from build123d import *

# Parameters (mm, degrees)
CROQUIS1_R              = 100
SALIENTE_EXTRUIR1_DEPTH = 3
CROQUIS3_R              = 110
CORTAR_EXTRUIR1_DEPTH   = 3
REDONDEO1_R             = 10
CORTAR_EXTRUIR2_DEPTH   = 142.453172607
CROQUIS5_R              = 1.5
CORTAR_EXTRUIR3_DEPTH   = 10
CROQUIS6_R              = 2
CORTAR_EXTRUIR4_DEPTH   = 142.453172607


with BuildPart() as part:
    # Croquis1 → Saliente-Extruir1 (new body)
    with BuildSketch(Plane.XY):
        Circle(CROQUIS1_R)
    extrude(amount=SALIENTE_EXTRUIR1_DEPTH)

    # Croquis3 → Cortar-Extruir1 (cut)
    with BuildSketch(Plane.XY.offset(3)):
        with Locations((190, 0)):
            Circle(CROQUIS3_R)
    extrude(amount=-CORTAR_EXTRUIR1_DEPTH, mode=Mode.SUBTRACT)

    # Redondeo1
    redondeo1_edges = [part.edges().sort_by_distance(p)[0] for p in [
        (89.473684211, -44.659375654, 1.5),
        (89.473684211, 44.659375654, 1.5),
    ]]
    fillet(redondeo1_edges, radius=REDONDEO1_R)

    # Croquis4 → Cortar-Extruir2 (cut, through all)
    with BuildSketch(Plane.XY.offset(3)):
        Polygon((-83.792153571, -57.629202667), (-57.629202667, -83.792153571), (-42.072853481, -68.235804385), (-45.290189335, -65.01846853), (-8.520636713, -28.248915908), (-28.248915908, -8.520636713), (-65.01846853, -45.290189335), (-68.235804385, -42.072853481), align=None)
        Polygon((-8.520636713, 31.077343033), (-28.248915908, 11.349063838), (-65.01846853, 48.11861646), (-68.235804385, 44.901280605), (-83.792153571, 60.457629791), (-57.629202667, 86.620580695), (-42.072853481, 71.064231509), (-45.290189335, 67.846895655), align=None)
        Polygon((31.077343033, 11.349063838), (11.349063838, 31.077343033), (48.11861646, 67.846895655), (44.901280605, 71.064231509), (60.457629791, 86.620580695), (86.620580695, 60.457629791), (71.064231509, 44.901280605), (67.846895655, 48.11861646), align=None)
        Polygon((11.349063838, -28.248915908), (31.077343033, -8.520636713), (67.846895655, -45.290189335), (71.064231509, -42.072853481), (86.620580695, -57.629202667), (60.457629791, -83.792153571), (44.901280605, -68.235804385), (48.11861646, -65.01846853), align=None)
    extrude(amount=-CORTAR_EXTRUIR2_DEPTH, mode=Mode.SUBTRACT)

    # Croquis5 → Cortar-Extruir3 (cut)
    with BuildSketch(Plane.XY.offset(3)):
        with Locations((-64.311361749, -40.340441867)):
            Circle(CROQUIS5_R)
        with Locations((-48.401459172, -24.43053929)):
            Circle(CROQUIS5_R)
        with Locations((-24.43053929, -48.401459172)):
            Circle(CROQUIS5_R)
        with Locations((-40.340441867, -64.311361749)):
            Circle(CROQUIS5_R)
        with Locations((-24.43053929, 51.229886297)):
            Circle(CROQUIS5_R)
        with Locations((-40.340441867, 67.139788874)):
            Circle(CROQUIS5_R)
        with Locations((-48.401459172, 27.258966415)):
            Circle(CROQUIS5_R)
        with Locations((-64.311361749, 43.168868991)):
            Circle(CROQUIS5_R)
        with Locations((51.229886297, 27.258966415)):
            Circle(CROQUIS5_R)
        with Locations((67.139788874, 43.168868991)):
            Circle(CROQUIS5_R)
        with Locations((27.258966415, 51.229886297)):
            Circle(CROQUIS5_R)
        with Locations((43.168868991, 67.139788874)):
            Circle(CROQUIS5_R)
        with Locations((27.258966415, -48.401459172)):
            Circle(CROQUIS5_R)
        with Locations((43.168868991, -64.311361749)):
            Circle(CROQUIS5_R)
        with Locations((51.229886297, -24.43053929)):
            Circle(CROQUIS5_R)
        with Locations((67.139788874, -40.340441867)):
            Circle(CROQUIS5_R)
    extrude(amount=-CORTAR_EXTRUIR3_DEPTH, mode=Mode.SUBTRACT)

    # Croquis6 → Cortar-Extruir4 (cut, through all)
    with BuildSketch(Plane(origin=(0, 0, 0), x_dir=(-1, 0, 0), z_dir=(0, 0, -1))):
        with Locations((-36.071652756, 84.633538668)):
            Circle(CROQUIS6_R)
        with Locations((34.338438835, 85.35145938)):
            Circle(CROQUIS6_R)
        with Locations((84.633538668, 36.071652756)):
            Circle(CROQUIS6_R)
        with Locations((85.35145938, -34.338438835)):
            Circle(CROQUIS6_R)
        with Locations((36.071652756, -84.633538668)):
            Circle(CROQUIS6_R)
        with Locations((-34.338438835, -85.35145938)):
            Circle(CROQUIS6_R)
    extrude(amount=-CORTAR_EXTRUIR4_DEPTH, mode=Mode.SUBTRACT)


solid = part.part
The listing builds one solid part. Answer for the finished solid, in the listing's coordinates (mm). A direction names the side the tool comes from. Coordinates: 2 decimals unless noted, no trailing zeros. Loops run counter-clockwise (first coordinate to the right, second up) from the corner with the lowest first, then second, coordinate; pieces in that order, holes last. Notation, with made-up numbers: (40, -9) -> (89, -9) arc R11 ccw to (89, 0) -> close; hole circle Ø9 at (-30, 73). An arc over 180 degrees is marked (long way). Write item = value, one per line. Start each with the question number.
1) A tool of negligible diameter and unlimited length cuts with its end or side. For faces 4 (the face through (-46.38, -26.65, 1.52)), 5 (the face through (-75.303, -49.14, 1.521)), 6 (the face through (-74.73, 51.396, 1.521)), from which of +Z, -Z, +X, -X, +Y, -Y can it reach the whole face along a straight path? Write none if from no direction.
2) Straight lines are drawn through the part: line 1 (X direction, y = 11.5, z = 2.05); line 2 (Y direction, x = 14, z = 1); line 3 (Y direction, x = 31.5, z = 2.7). For each, find the intervals that lie inside material, in ascending order. Write a range as from..to.
3) A cutting plane is placed at D-D (y = -1.5). Give the vertices of the cut face in (x, z).
4) A cutting plane is placed at A-A (x = 14). Give the vertices of the cut face in (y, z), then the cut area to 3 significant figures.
5) A cutting plane is placed at C-C (z = 2.3). Count the separate pieces of the cut face and the enclosed holes in it, then the cut area to 3 significant figures.
6) The mould has two halves that part along X. Classify faces 1 (the face through (84.96, 52.74, 1.48)), 2 (the face through (-99.983, 1.869, 1.479)), 3 (the face through (29.476, 49.205, 1.521)): released by +X, released by -X, zero draft, split by the parting line, or undercut.
7) A cutting plane is placed at B-B (y = -60). Give the vertices of the cut face in (x, z).
Responses:
q1.face_4 = +Z, -Z
q1.face_5 = +Z, -Z, -Y
q1.face_6 = +Z, -Z, +Y
q2.line_1 = -99.34..-28.4, -28.1..30.93, 31.23..80.6
q2.line_2 = -99.02..-30.9, -25.6..28.43, 33.73..99.02
q2.line_3 = -94.91..-48.4, -8.94..11.77, 51.23..94.91
q3.outline = (-99.99, 0) -> (80.01, 0) -> (80.01, 3) -> (-99.99, 3) -> close
q4.outline = (-99.02, 0) -> (-30.9, 0) -> (-30.9, 3) -> (-99.02, 3) -> close; (-25.6, 0) -> (28.43, 0) -> (28.43, 3) -> (-25.6, 3) -> close; (33.73, 0) -> (99.02, 0) -> (99.02, 3) -> (33.73, 3) -> close
q4.area = 562 mm²
q5.separate_pieces = 1
q5.enclosed_holes = 22
q5.area = 21,300 mm²
q6.face_1 = released by +X
q6.face_2 = released by -X
q6.face_3 = undercut
q7.outline = (-40.27, 0) -> (43.1, 0) -> (43.1, 3) -> (-40.27, 3) -> close
